from build123d import *

# Parameters (mm, degrees)
SKETCH1_R           = 4.1656
BOSS_EXTRUDE1_DEPTH = 6.35


with BuildPart() as part:
    # Sketch1 → Boss-Extrude1 (new body)
    with BuildSketch(Plane.XY.offset(6.35)):
        Polygon((-19.05, 152.4), (-76.2, 38.1), (-76.2, 0), (76.2, 0), (76.2, 38.1), (19.05, 152.4), align=None)
        with Locations((-57.15, 19.05)):
            Circle(SKETCH1_R, mode=Mode.SUBTRACT)
        with Locations((-19.05, 19.05)):
            Circle(SKETCH1_R, mode=Mode.SUBTRACT)
        with Locations((0, 133.35)):
            Circle(SKETCH1_R, mode=Mode.SUBTRACT)
        with Locations((0, 95.25)):
            Circle(SKETCH1_R, mode=Mode.SUBTRACT)
        with Locations((0, 57.15)):
            Circle(SKETCH1_R, mode=Mode.SUBTRACT)
        with Locations((19.05, 19.05)):
            Circle(SKETCH1_R, mode=Mode.SUBTRACT)
        with Locations((57.15, 19.05)):
            Circle(SKETCH1_R, mode=Mode.SUBTRACT)
    extrude(amount=-BOSS_EXTRUDE1_DEPTH)


solid = part.part
Can you work these out from the model? Positions are in its coordinate system, mm. Give positions to 0.01 mm unless a question says otherwise; leave off trailing zeros. Order: outer loops, then holes, each group sorted by start corner. A loop starts at its lowest first (then second) coordinate and runs counter-clockwise, first axis right, second up. Notation, with made-up numbers: M -22,77 L 36,77 A24 ccw 36,100 Z; hole C 88.5,48.25 d8. An arc over 180 degrees is marked long. Use one line per item in the form item = value. Start each with the question number.
Item 1: If we section it at D-D (x = 0): Write out the boundary of the cut face in (y, z).
Item 2: If we section it at C-C (z = 2.25): Write out the boundary of the cut face in (x, y), then the cut area to 3 significant figures.
Item 3: If we section it at B-B (x = -57.15): Write out the boundary of the cut face in (y, z), then the cut area to 3 significant figures.
Item 4: If I drill on line 1 along Y through (x, z) = (57.15, 4); line 2 along Y through (x, z) = (0, 4.5); line 3 along X through (y, z) = (129.5, 1.25), over which ranges is the centre line in solid material (lowest first)?
Item 5: Will these pins go through, and if not, where does the flat tip stop? pin 1 Ø2 at (y, z) = (65, 1) entering from +X; pin 2 Ø2 at (y, z) = (82.5, 0.5) entering from -X; pin 3 Ø1 at (x, z) = (47.5, 3.5) entering from +Y.
Item 6: If we section it at A-A (y = 19.05): Write out the boundary of the cut face in (x, z).
Item 7: We'd pull the mould along Y, two halves only. Please class faces 1 (the cylindrical face through (53.84, 16.52, 3.22)), 2 (the flat face through (-76.2, 19, 3)), 3 (the flat face through (-47.2, 96.1, 3.2)): +Y half, -Y half, draft (parallel to the pull), parting line (faces both ways), or undercut.
Outcome:
q1.outline = M 0,0 L 52.98,0 L 52.98,6.35 L 0,6.35 Z; M 61.32,0 L 91.08,0 L 91.08,6.35 L 61.32,6.35 Z; M 99.42,0 L 129.18,0 L 129.18,6.35 L 99.42,6.35 Z; M 137.52,0 L 152.4,0 L 152.4,6.35 L 137.52,6.35 Z
q2.outline = M -76.2,0 L 76.2,0 L 76.2,38.1 L 19.05,152.4 L -19.05,152.4 L -76.2,38.1 Z; hole C -57.15,19.05 d8.33; hole C -19.05,19.05 d8.33; hole C 0,57.15 d8.33; hole C 0,95.25 d8.33; hole C 0,133.35 d8.33; hole C 19.05,19.05 d8.33; hole C 57.15,19.05 d8.33
q2.area = 16,300 mm2
q3.outline = M 0,0 L 14.88,0 L 14.88,6.35 L 0,6.35 Z; M 23.22,0 L 76.2,0 L 76.2,6.35 L 23.22,6.35 Z
q3.area = 431 mm2
q4.line_1 = 0 to 14.88, 23.22 to 76.2
q4.line_2 = 0 to 52.98, 61.32 to 91.08, 99.42 to 129.18, 137.52 to 152.4
q4.line_3 = -30.5 to -1.59, 1.59 to 30.5
q5.pin_1 = 63.25
q5.pin_2 = -54.5
q5.pin_3 = 96.5
q6.outline = M -76.2,0 L -61.32,0 L -61.32,6.35 L -76.2,6.35 Z; M -52.98,0 L -23.22,0 L -23.22,6.35 L -52.98,6.35 Z; M -14.88,0 L 14.88,0 L 14.88,6.35 L -14.88,6.35 Z; M 23.22,0 L 52.98,0 L 52.98,6.35 L 23.22,6.35 Z; M 61.32,0 L 76.2,0 L 76.2,6.35 L 61.32,6.35 Z
q7.face_1 = undercut
q7.face_2 = draft
q7.face_3 = +Y half
